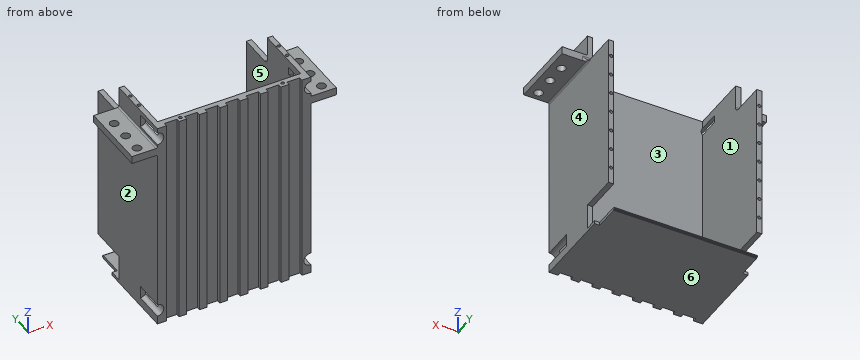
from build123d import *

# Parameters (mm, degrees)
BASE_DEPTH         = 52.831999999999994
BATTERY_HOLE_DEPTH = 48.4251
EXTRUDE3_DEPTH     = 52.831999999999994
FILLET1_R          = 0.762
SKETCH6_W          = 6.350000000000001
SKETCH6_H          = 1.904999999999987
SKETCH6_W_2        = 6.349999999999994
EXTRUDE5_DEPTH     = 106.3625
SKETCH5_R          = 0.812800000000009
SKETCH5_R_2        = 0.8128000000000078
SKETCH5_R_3        = 0.812799999999968
EXTRUDE6_DEPTH     = 9.525
SKETCH10_R         = 3.1749999999999976
SKETCH10_R_2       = 3.1750000000000003
EXTRUDE8_DEPTH     = 15.239999999999998
SKETCH12_W         = 14.28749999999998
SKETCH12_H         = 18.795999999999985
EXTRUDE9_DEPTH     = 157.4558690054483
SKETCH13_R         = 0.8128000000000039
SKETCH13_R_2       = 0.8128000000000078
SKETCH13_R_3       = 0.812800000000012
EXTRUDE10_DEPTH    = 10
SKETCH16_R         = 3.174999999999997
EXTRUDE13_DEPTH    = 15.239999999999998
SKETCH17_W         = 76.454
SKETCH17_H         = 1.5747999999999962
EXTRUDE14_DEPTH    = 6.35
SKETCH19_R         = 2.158999999999993
SKETCH19_R_2       = 2.159
SKETCH19_R_3       = 2.158999999999994
EXTRUDE15_DEPTH    = 14.2875
SKETCH20_R         = 0.8128000000000078
SKETCH20_R_2       = 0.8127999999999996
EXTRUDE16_DEPTH    = 9.525
SKETCH22_W         = 71.2978
SKETCH22_H         = 1.5747999999999962
EXTRUDE17_DEPTH    = 12.446
SKETCH24_W         = 5.020847259377149
SKETCH24_H         = 12.98126293619711
SKETCH24_W_2       = 5.020847259377153
SKETCH24_H_2       = 12.9812629361971
EXTRUDE18_DEPTH    = 18.796
FILLET2_R          = 2.54
SKETCH25_W         = 71.29779999999998
SKETCH25_H         = 0.6667500000000075
EXTRUDE19_DEPTH    = 0.79375
CHAMFER1_SIZE      = 0.1778


with BuildPart() as part:
    # Sketch1 → base (new body)
    with BuildSketch(Plane(origin=(0, 0, 0), x_dir=(1, 0, 0), z_dir=(0, 1, 0))):
        Polygon((0, 0), (-76.454, 4.51e-15), (-76.454, 106.3625), (0, 106.3625), align=None)
    extrude(amount=-BASE_DEPTH)

    # Sketch2 → battery hole (cut)
    with BuildSketch(Plane(origin=(0, 0, 0), x_dir=(1, 0, 0), z_dir=(0, 1, 0))):
        Polygon((-73.8759, 104.78769999999999), (-2.5781000000000067, 104.78769999999999), (-2.578100000000014, 0), (-73.87589999999999, 0), align=None)
    extrude(amount=-BATTERY_HOLE_DEPTH, mode=Mode.SUBTRACT)

    # Sketch4 → Extrude3 (add)
    with BuildSketch(Plane(origin=(0, 0, 0), x_dir=(-1, 0, 0), z_dir=(0, 1, 0))):
        Polygon((76.45400000000001, -14.287499999999994), (89.154, -14.287499999999994), (89.154, -10.477499999999996), (76.45400000000001, -10.477499999999997), align=None)
        Polygon((0, -10.477499999999997), (0, -14.287499999999994), (-12.699999999999989, -14.287499999999994), (-12.699999999999989, -10.477499999999996), align=None)
    extrude(amount=-EXTRUDE3_DEPTH)

    # Fillet1
    fillet1_edges = [part.edges().sort_by_distance(p)[0] for p in [
        (0, -26.415999999999997, -14.287499999999994),
        (-76.45400000000001, -26.415999999999997, -14.287499999999994),
        (0, -26.415999999999997, -10.477499999999997),
        (-76.45400000000001, -26.415999999999997, -10.477499999999997),
    ]]
    fillet(fillet1_edges, radius=FILLET1_R)

    # Sketch6 → Extrude5 (cut)
    with BuildSketch(Plane.XY):
        with Locations((-58.68648014601246, -51.8795)):
            Rectangle(SKETCH6_W, SKETCH6_H)
        with Locations((-48.526480146012446, -51.8795)):
            Rectangle(SKETCH6_W_2, SKETCH6_H)
        with Locations((-38.366480146012435, -51.8795)):
            Rectangle(SKETCH6_W_2, SKETCH6_H)
        with Locations((-28.20648014601243, -51.8795)):
            Rectangle(SKETCH6_W_2, SKETCH6_H)
        with Locations((-18.046480146012428, -51.8795)):
            Rectangle(SKETCH6_W_2, SKETCH6_H)
        with Locations((-7.60751985398754, -51.8795)):
            Rectangle(SKETCH6_W_2, SKETCH6_H)
        with Locations((-68.84648014601245, -51.8795)):
            Rectangle(SKETCH6_W_2, SKETCH6_H)
    extrude(amount=-EXTRUDE5_DEPTH, mode=Mode.SUBTRACT)

    # Sketch5 → Extrude6 (cut)
    with BuildSketch(Plane.XY):
        with Locations((-75.16494999999998, -26.415999999999993)):
            Circle(SKETCH5_R)
        with Locations((-75.16494999999985, -34.03599999999999)):
            Circle(SKETCH5_R_2)
        with Locations((-1.289050000000194, -34.035999999999994)):
            Circle(SKETCH5_R_3)
        with Locations((-1.2890500000000276, -26.415999999999997)):
            Circle(SKETCH5_R)
    extrude(amount=-EXTRUDE6_DEPTH, mode=Mode.SUBTRACT)

    # Sketch10 → Extrude8 (cut)
    with BuildSketch(Plane.XZ.offset(52.831999999999994)):
        with Locations((-76.454, -5.587999999999997)):
            Circle(SKETCH10_R)
        with Locations((0, -5.587999999999997)):
            Circle(SKETCH10_R_2)
    extrude(amount=-EXTRUDE8_DEPTH, mode=Mode.SUBTRACT)

    # Sketch12 → Extrude9 (cut, through all)
    with BuildSketch(Plane(origin=(12.699999999999989, 0, 0), x_dir=(0, 0, -1), z_dir=(1, 0, 0))):
        Polygon((0, 0), (14.287499999999994, 0), (14.287499999999994, -18.796), (2.3e-15, -18.796), align=None)
        with Locations((99.21875, -9.397999999999993)):
            Rectangle(SKETCH12_W, SKETCH12_H)
    extrude(amount=-EXTRUDE9_DEPTH, mode=Mode.SUBTRACT)

    # Sketch13 → Extrude10 (cut)
    with BuildSketch(Plane(origin=(0, 0, 0), x_dir=(-1, 0, 0), z_dir=(0, 1, 0))):
        with Locations(Location((75.16495000000032, -83.66125, 0), (0, 0, 90))):
            Circle(SKETCH13_R)
        with Locations(Location((75.1649500000002, -73.50125, 0), (0, 0, 90))):
            Circle(SKETCH13_R_2)
        with Locations(Location((75.16494999999995, -43.021249999999995, 0), (0, 0, 90))):
            Circle(SKETCH13_R_2)
        with Locations(Location((1.289050000000111, -22.701249999999998, 0), (0, 0, 90))):
            Circle(SKETCH13_R_2)
        with Locations(Location((1.2890499999996945, -83.66125, 0), (0, 0, 90))):
            Circle(SKETCH13_R)
        with Locations(Location((1.2890499999998055, -73.50125000000001, 0), (0, 0, 90))):
            Circle(SKETCH13_R_3)
        with Locations(Location((75.1649500000001, -63.34125, 0), (0, 0, 90))):
            Circle(SKETCH13_R_2)
        with Locations(Location((75.16494999999999, -53.18125, 0), (0, 0, 90))):
            Circle(SKETCH13_R_2)
        with Locations(Location((75.16494999999992, -32.86124999999999, 0), (0, 0, 90))):
            Circle(SKETCH13_R_2)
        with Locations(Location((75.16494999999988, -22.701249999999998, 0), (0, 0, 90))):
            Circle(SKETCH13_R_2)
        with Locations(Location((1.2890500000000693, -32.86124999999999, 0), (0, 0, 270))):
            Circle(SKETCH13_R_2)
        with Locations(Location((1.2890500000000416, -43.021249999999995, 0), (0, 0, 270))):
            Circle(SKETCH13_R_2)
        with Locations(Location((1.2890500000000138, -53.18125, 0), (0, 0, 270))):
            Circle(SKETCH13_R_2)
        with Locations(Location((1.2890499999999028, -63.34125, 0), (0, 0, 270))):
            Circle(SKETCH13_R_2)
    extrude(amount=-EXTRUDE10_DEPTH, mode=Mode.SUBTRACT)

    # Sketch16 → Extrude13 (cut)
    with BuildSketch(Plane.XZ.offset(52.831999999999994)):
        with Locations((-76.454, -98.9965)):
            Circle(SKETCH16_R)
        with Locations((-0.27896029202487127, -98.9965)):
            Circle(SKETCH16_R)
    extrude(amount=-EXTRUDE13_DEPTH, mode=Mode.SUBTRACT)

    # Sketch17 → Extrude14 (add)
    with BuildSketch(Plane(origin=(0, -18.795999999999985, 0), x_dir=(1, 0, 0), z_dir=(0, 1, 0))):
        with Locations((-38.227, 105.57509999999999)):
            Rectangle(SKETCH17_W, SKETCH17_H)
    extrude(amount=EXTRUDE14_DEPTH)

    # Sketch19 → Extrude15 (cut)
    with BuildSketch(Plane.XY):
        with Locations((-84.201, -48.513999999999996)):
            Circle(SKETCH19_R)
        with Locations((-84.201, -38.35399999999999)):
            Circle(SKETCH19_R)
        with Locations((7.747000000000003, -48.513999999999996)):
            Circle(SKETCH19_R_2)
        with Locations((7.747000000000003, -38.35399999999999)):
            Circle(SKETCH19_R_2)
        with Locations((-84.201, -28.19399999999999)):
            Circle(SKETCH19_R_3)
        with Locations((7.747000000000003, -28.19399999999999)):
            Circle(SKETCH19_R_3)
    extrude(amount=-EXTRUDE15_DEPTH, mode=Mode.SUBTRACT)

    # Sketch20 → Extrude16 (cut)
    with BuildSketch(Plane.XY):
        with Locations((-63.766480146012455, -50.62855)):
            Circle(SKETCH20_R)
        with Locations((-12.826999999999984, -50.62855)):
            Circle(SKETCH20_R_2)
    extrude(amount=-EXTRUDE16_DEPTH, mode=Mode.SUBTRACT)

    # Sketch22 → Extrude17 (add)
    with BuildSketch(Plane(origin=(0, -12.445999999999987, 0), x_dir=(1, 0, 0), z_dir=(0, 1, 0))):
        with Locations((-38.227000000000004, 105.57509999999999)):
            Rectangle(SKETCH22_W, SKETCH22_H)
    extrude(amount=EXTRUDE17_DEPTH)

    # Sketch24 → Extrude18 (cut)
    with BuildSketch(Plane(origin=(0, 0, 0), x_dir=(1, 0, 0), z_dir=(0, 1, 0))):
        with Locations((-78.96442362968857, 11.223602435904425)):
            Rectangle(SKETCH24_W, SKETCH24_H)
        with Locations((2.5104236296885767, 11.223602435904418)):
            Rectangle(SKETCH24_W_2, SKETCH24_H_2)
    extrude(amount=-EXTRUDE18_DEPTH, mode=Mode.SUBTRACT)

    # Fillet2
    fillet2_edges = [part.edges().sort_by_distance(p)[0] for p in [
        (-1.2890500000000067, -18.796, -14.287499999999994),
        (-75.16494999999999, -18.796, -14.287499999999994),
        (-76.454, -18.796, -14.668499999999995),
        (0, -18.796, -14.668499999999995),
    ]]
    fillet(fillet2_edges, radius=FILLET2_R)

    # Sketch25 → Extrude19 (add)
    with BuildSketch(Plane(origin=(0, 0, 0), x_dir=(1, 0, 0), z_dir=(0, 1, 0))):
        with Locations((-38.227, 105.57509999999996)):
            Rectangle(SKETCH25_W, SKETCH25_H)
    extrude(amount=EXTRUDE19_DEPTH)

    # Chamfer1
    chamfer1_edges = [part.edges().sort_by_distance(p)[0] for p in [
        (-38.227, 0.79375, -105.90847499999997),
        (-38.227, 0.79375, -105.24172499999997),
        (-38.227, 0, -105.24172499999997),
        (-38.227, 0, -105.90847499999997),
    ]]
    chamfer(chamfer1_edges, length=CHAMFER1_SIZE)


solid = part.part
Build history of the part. All positions in model axes, mm. Face numbers are marked on the shaded views. A direction names the side the tool comes from. Coordinates: 2 decimals unless noted, no trailing zeros. Write each loop counter-clockwise with the first axis right and the second up, starting at its lowest first coordinate (ties: lowest second). Pieces come first, ordered by that corner, then holes.
(1) Mould opens along X. For the marked faces 1, 2, 3 and 4 say: pulls with the +X half, pulls with the -X half, needs draft (parallel to the pull), parting line crosses it, or undercut.
(2) 3-axis set-ups, long thin cutter, end or side, ignore diameter. For the marked faces 5 and 6: which of +Z, -Z, +X, -X, +Y, -Y reach the whole face in a straight line?
(3) Cut at B-B on x = -67.5. List the corners of the cut face in (y, z), and give its area (3 significant figures).
(4) Pin check, flat tips, straight feed: pin 1 Ø7 at (x, z) = (-83.5, -7.5) entering from +Y; pin 2 Ø1.8 at (x, z) = (-1.5, -43) entering from +Y; pin 3 Ø6 at (y, z) = (-23, -45) entering from +X; pin 4 Ø13 at (x, y) = (4, -41.5) entering from +Z. Stop position of each tip, or through.
(5) Cut at A-A on x = -44. List the corners of the cut face in (y, z).
(6) Drill centre lines: line 1 (X direction, y = -23, z = -35); line 2 (Z direction, x = -76, y = -43); line 3 (Y direction, x = -57.5, z = -70.5). Where is each one in solid material? Low to high.
Working result:
1. face 1: undercut
1. face 2: pulls with the -X half
1. face 3: undercut
1. face 4: pulls with the +X half
2. face 5: +Z, +Y
2. face 6: -Z, +X, -X, +Y, -Y
3. outline: (-50.93, -106.36) - (0, -106.36) - (0, -106.09) - (0.18, -105.91) - (0.62, -105.91) - (0.79, -105.73) - (0.79, -105.42) - (0.62, -105.24) - (0.18, -105.24) - (0, -105.06) - (0, -104.79) - (-48.43, -104.79) - (-48.43, 0) - (-50.93, 0) - close
3. area: 343 mm2
4. pin 1: stops at y = -18.8
4. pin 2: stops at y = 0
4. pin 3: stops at x = 0
4. pin 4: stops at z = 0
5. outline: (-52.83, -106.36) - (0, -106.36) - (0, -106.09) - (0.18, -105.91) - (0.62, -105.91) - (0.79, -105.73) - (0.79, -105.42) - (0.62, -105.24) - (0.18, -105.24) - (0, -105.06) - (0, -104.79) - (-48.43, -104.79) - (-48.43, 0) - (-52.83, 0) - close
6. line 1: x = -76.45 to -73.88, -2.58 to 0
6. line 2: z = -106.36 to -102.14, -95.85 to -8.73, -2.45 to 0
6. line 3: y = -50.93 to -48.43
